Autodesk Fusion 360 part; units mm, degrees
sketch "Sketch1" plane through (0, 0, 0) normal (0, 0, 1) x (1, 0, 0)
  line L0 (-221.214, 50) -> (125, 50)
  line L1 (125, 50) -> (125, -80.212)
  line L2 (125, -80.212) -> (-221.214, -80.212)
  line L3 (-221.214, -80.212) -> (-221.214, 50)
  line L4 (-231.214, 60) -> (135, 60)
  line L5 (135, 60) -> (135, -90.212)
  line L6 (135, -90.212) -> (-231.214, -90.212)
  line L7 (-231.214, -90.212) -> (-231.214, 60)
  circle A0 centre (-225.714, 54.5) radius 1.45
  circle A1 centre (129.5, 54.5) radius 1.45
  circle A2 centre (129.5, -84.712) radius 1.45
  circle A3 centre (-225.714, -84.712) radius 1.45
  dimension "d1" = 130.212
  dimension "d2" = 346.214
  dimension "d3" = 10
  dimension "d4" = 10
  dimension "d5" = 10
  dimension "d6" = 10
  dimension "d15" = 2.9
  dimension "d16" = 5.5
  dimension "d17" = 5.5
  dimension "d18" = 2.9
  dimension "d19" = 5.5
  dimension "d20" = 5.5
  dimension "d21" = 2.9
  dimension "d22" = 5.5
  dimension "d23" = 5.5
  dimension "d24" = 2.9
  dimension "d25" = 5.5
  dimension "d26" = 5.5
extrude "Extrude1" add sketch "Sketch1" along normal blind 3 contours L0 L1 L2 L3
extrude "Extrude2" add sketch "Sketch1" along normal blind 13 contours L4 L5 L6 L7 | A0 | A1 | A2 | A3
sketch "Sketch3" plane through (0, 60, 0) normal (0, 1, 0) x (-1, 0, 0)
  line L0 (-135, 0) -> (231.214, 0)
  line L1 (231.214, 0) -> (231.214, 13)
  line L2 (231.214, 13) -> (-135, 13)
  line L3 (-135, 13) -> (-135, 0)
  line L4 (-117.016, 13) -> (-93.016, 13)
  line L5 (-93.016, 13) -> (-93.016, 2)
  line L6 (-93.016, 2) -> (-117.016, 2)
  line L7 (-117.016, 2) -> (-117.016, 13)
  dimension "d11" = 24
  dimension "d12" = 17.984
extrude "Extrude3" cut sketch "Sketch3" against normal blind 10 contours L2 L4 L5 L6 L7
extrude "Extrude4" cut sketch "Sketch1" along normal blind 13 contours A0 | A1 | A2 | A3
fillet "Fillet1" radius 7 4 edges at (135, -90.212, 6.5) (135, 60, 6.5) (-231.214, 60, 6.5) (-231.214, -90.212, 6.5)
Can you work these out from the model? Positions are in its coordinate system, mm. A direction names the side the tool comes from. Give positions to 0.01 mm unless a question says otherwise; leave off trailing zeros. Write each loop counter-clockwise with the first axis right and the second up, starting at its lowest first coordinate (ties: lowest second). Pieces come first, ordered by that corner, then holes. Notation, with made-up numbers: (21, 20.5) -> (39, 20.5) arc R27 cw to (39, 49.5) -> close; hole circle Ø8 at (51, 46). An arc over 180 degrees is marked (long way). One line per item, written item: value.
Q1. Imagine slicing it at A-A on y = 15. Please give me the cut outline in (x, z).
Results found:
outline: (-231.21, 0) -> (135, 0) -> (135, 13) -> (125, 13) -> (125, 3) -> (-221.21, 3) -> (-221.21, 13) -> (-231.21, 13) -> close
Q2. Imagine slicing it at B-B on z = 8.5. Please give me the cut outline in (x, y).
Results found:
outline: (-231.21, -83.21) arc R7 ccw to (-224.21, -90.21) -> (128, -90.21) arc R7 ccw to (135, -83.21) -> (135, 53) arc R7 ccw to (128, 60) -> (117.02, 60) -> (117.02, 50) -> (125, 50) -> (125, -80.21) -> (-221.21, -80.21) -> (-221.21, 50) -> (93.02, 50) -> (93.02, 60) -> (-224.21, 60) arc R7 ccw to (-231.21, 53) -> close; hole circle Ø2.9 at (-225.71, -84.71); hole circle Ø2.9 at (-225.71, 54.5); hole circle Ø2.9 at (129.5, -84.71); hole circle Ø2.9 at (129.5, 54.5)
Q3. Imagine slicing it at C-C on x = 75. Please give me the cut outline in (y, z), and give its area (3 significant figures).
Results found:
outline: (-90.21, 0) -> (60, 0) -> (60, 13) -> (50, 13) -> (50, 3) -> (-80.21, 3) -> (-80.21, 13) -> (-90.21, 13) -> close
area: 651 mm^2
Q4. Please list where these lines run through material, in increasing order: line 1 (Y direction, x = -84, z = 6); line 2 (X direction, y = 35, z = 4.75); line 3 (Y direction, x = 129.5, z = 7). Write a range as [from, to].
Results found:
line 1: y = [-90.21, -80.21], [50, 60]
line 2: x = [-231.21, -221.21], [125, 135]
line 3: y = [-90.05, -86.16], [-83.26, 53.05], [55.95, 59.84]
Q5. We'd pull the mould along X, two halves only. Please class faces 4 (the face through (-51, -14, 0)), 5 (the face through (135, -14, 6)), 6 (the face through (105, 55, 2)): +X half, -X half, draft (parallel to the pull), parting line (faces both ways), or undercut.
Results found:
face 4: draft
face 5: +X half
face 6: undercut
Q6. Which directions (+Z, -Z, +X, -X, +Y, -Y) give clear straight access to the entire face, cutting with the end or side of a thin tool? Please do faces 1 (the face through (-221.214, -16, 8)), 2 (the face through (-46, -90.212, 6)), 3 (the face through (93.016, 55, 8)).
Results found:
face 1: +Z
face 2: +Z, -Z, +X, -X, -Y
face 3: +Z, +Y
Q7. For P1, Ø2.5, axis at x = -225.714, y = 54.5, coming from the -Z side, with a flat end and sliding along its axis, tell me the tip position at first contact or that it passes through.
Results found:
P1: passes through
